from build123d import *

# Parameters (mm, degrees)
CROQUIS1_W              = 45
CROQUIS1_H              = 60
SALIENTE_EXTRUIR1_DEPTH = 7.5
CROQUIS2_W              = 4
CROQUIS2_H              = 170


with BuildPart() as part:
    # Croquis1 → Saliente-Extruir1 (new, symmetric)
    with BuildSketch(Plane.XY):
        Rectangle(CROQUIS1_W, CROQUIS1_H)
    extrude(amount=SALIENTE_EXTRUIR1_DEPTH, both=True)

    # Croquis2 → Revolución1 (revolve)
    with BuildSketch(Plane.XY, mode=Mode.PRIVATE) as revoluci_n1_sk:
        with Locations((-14, 115)):
            Rectangle(CROQUIS2_W, CROQUIS2_H)
    revoluci_n1 = revolve(revoluci_n1_sk.sketch.rotate(Axis((-12, 30, 0), (0, 1, 0)), 270), axis=Axis((-12, 30, 0), (0, 1, 0)))

    # Simetría1: Revolución1 across plane
    add(revoluci_n1.mirror(Plane(origin=(0, 0, 0), x_dir=(0, 0, 1), z_dir=(1, 0, 0))))


solid = part.part
For this review, take the finished solid that the model builds, in its own axes (mm). A direction names the side the tool comes from. Give positions to 0.01 mm unless a question says otherwise; leave off trailing zeros. Loops run counter-clockwise (first coordinate to the right, second up) from the corner with the lowest first, then second, coordinate; pieces in that order, holes last. Notation, with made-up numbers: M 86,87 L 113,87 A31 cw 113,119 Z; hole C -24,-38 d3. An arc over 180 degrees is marked long. Answer as a JSON object with one key per item and string values. Group by question number.
Q1. For probe 1 along X at (y, z) = (116, 0); probe 2 along Y at (x, z) = (-6, 6); probe 3 along X at (y, z) = (177.5, 2.75), list the stretches that pass through material, from the lowest coordinate up. Write a range as [from, to].
Q2. Mouldability with a two-part tool opening along X and no side actions: class faces 1 (the flat face through (-22.5, 0, 0)), 2 (the flat face through (0, 30, 0)), 3 (the flat face through (-12, 200, 0)), 4 (the cylindrical face through (15.966, 116.19, 0.521)) as +X half, -X half, draft (parallel to the pull), parting line (faces both ways), or undercut.
Q3. Insertion check: P1, Ø3, axis at y = 74, z = 4.5, coming from the -X side; P2, Ø3, axis at x = 5.5, y = 140, coming from the +Z side; P3, Ø5, axis at y = 107.5, z = 3, coming from the +X side. Each pin has a flat end and moves straight along its axis. Give the tip position at first contact, or say it passes through.
Q4. Tool access review of faces 5 (the flat face through (12, 200, 0)), 6 (the cylindrical face through (-15.966, 116.19, 0.521)): name each direction out of +Z, -Z, +X, -X, +Y, -Y from which nothing blocks a thin tool from reaching the whole face with its end or side.
Q5. Add section B-B on x = -12. Give the boundary of the cut face in (y, z), and give its area (3 significant figures).
Q6. Add section C-C on y = 97. Give the boundary of the cut face in (x, z).
Q7. Add section A-A on z = 0. Give the boundary of the cut face in (x, y), and give its area (3 significant figures).
Q8. Add section D-D on x = -2. Give the boundary of the cut face in (y, z).
Checked values:
{
 "1": {"probe 1": "[-16, -8], [8, 16]", "probe 2": "[-30, 30]", "probe 3": "[-14.9, -9.1], [9.1, 14.9]"},
 "2": {"face 1": "-X half", "face 2": "undercut", "face 3": "draft", "face 4": "undercut"},
 "3": {"P1": "x = -14.65", "P2": "through", "P3": "x = 15.97"},
 "4": {"face 5": "+Z, -Z, +X, -X, +Y", "face 6": "+Y"},
 "5": {"outline": "M -30,-7.5 L 30,-7.5 L 30,-4 L 200,-4 L 200,4 L 30,4 L 30,7.5 L -30,7.5 Z", "area": "2,260 mm²"},
 "6": {"outline": "C -12,0 d8; C 12,0 d8"},
 "7": {"outline": "M -22.5,-30 L 22.5,-30 L 22.5,30 L 16,30 L 16,200 L 8,200 L 8,30 L -8,30 L -8,200 L -16,200 L -16,30 L -22.5,30 Z", "area": "5,420 mm²"},
 "8": {"outline": "M -30,-7.5 L 30,-7.5 L 30,7.5 L -30,7.5 Z"}
}
